The model under review builds one solid part; all positions refer to its coordinate system, in mm. Face numbers are marked on the shaded views. Round coordinates to 2 decimals unless told otherwise and drop trailing zeros. Write each loop counter-clockwise with the first axis right and the second up, starting at its lowest first coordinate (ties: lowest second). Pieces come first, ordered by that corner, then holes. Notation, with made-up numbers: (5, 11) -> (50, 11) arc R19 ccw to (50, 15) -> close; hole circle Ø7 at (-20, 89.25). An arc over 180 degrees is marked (long way). Answer in a Markdown table with one row per item. Add a question column.
```python
from build123d import *

# Parameters (mm, degrees)
F2_R = 10
F3_R = 5


with BuildPart() as f1:
    # F0 (on Front) → F1 (revolve)
    with BuildSketch(Plane.XZ):
        Polygon((14, 30), (0, 30), (0, -30), (14, -30), (14, -25), (4, -15), (4, 0), (4, 15), (14, 25), align=None)
    revolve(axis=Axis((0, 0, 0), (0, 0, -1)))

    # F2
    f2_edges = [f1.edges().sort_by_distance(p)[0] for p in [
        (-4, 0, 15),
        (-4, 0, -15),
    ]]
    fillet(f2_edges, radius=F2_R)

    # F3
    f3_edges = [f1.edges().sort_by_distance(p)[0] for p in [
        (-14, 0, 25),
        (-14, 0, -25),
    ]]
    fillet(f3_edges, radius=F3_R)


solid = f1.part
```
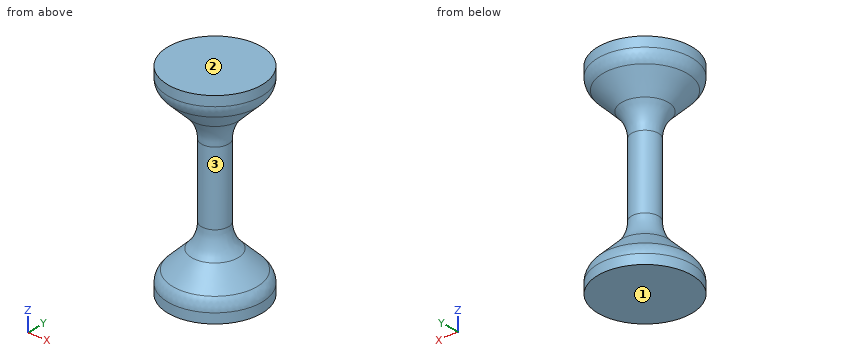
1. For L1, parallel to Z at x = 5.75, y = -2.75; L2, parallel to Z at x = -10, y = -3.5; L3, parallel to X at y = 9, z = 23.5, list the stretches that pass through material, from the lowest coordinate up.
2. Add section A-A on z = 8.5. Write out the cut boundary in (x, y).
3. Mouldability with a two-part tool opening along Z and no side actions: class the marked faces 1, 2 and 3 as pulls with the +Z half, pulls with the -Z half, needs draft (parallel to the pull), parting line crosses it, or undercut.
4. Insertion check: pin 1 Ø4 at (x, z) = (-4, -0.5) entering from -Y. The pin has a flat end and moves straight along its axis. Give the tip position at first contact, or say it passes through.
Filled in:
| question | item | result |
|---|---|---|
| 1 | L1 | -30 to -17.33, 17.33 to 30 |
| 1 | L2 | -30 to -21.59, 21.59 to 30 |
| 1 | L3 | -8.67 to 8.67 |
| 2 | outline | circle Ø8 at (0, 0) |
| 3 | face 1 | pulls with the -Z half |
| 3 | face 2 | pulls with the +Z half |
| 3 | face 3 | undercut |
| 4 | pin 1 | y = -3.46 |
